Geometry: final body of the model. Coordinates: model frame, mm. Face numbers are marked on the shaded views. A direction names the side the tool comes from. Give positions to 0.01 mm unless a question says otherwise; leave off trailing zeros. Write each loop counter-clockwise with the first axis right and the second up, starting at its lowest first coordinate (ties: lowest second). Pieces come first, ordered by that corner, then holes. Notation, with made-up numbers: (-19.75, -23) -> (-9.75, -23) arc R11 ccw to (-9.75, -18) -> close; hole circle Ø4 at (59, 16.25). An arc over 180 degrees is marked (long way). Answer in a Markdown table with one row per item. Add a question column.
Item 1: Section query C-C on z = -28.5. Output: boundary loops of the cut face in (x, y).
Item 2: First-contact query: P1, Ø0.7, axis at x = -24.5, y = -7, coming from the +Z side; P2, Ø3, axis at x = -11.5, y = 2.5, coming from the -Z side; P3, Ø2, axis at x = 8, z = -39.5, coming from the +Y side. Flat tips, straight axial feed; report the tip coordinate or a pass-through.
Item 3: Material intervals for probe 1 along Y at (x, z) = (-13, -43); probe 2 along Z at (x, y) = (0, -6.25); probe 3 along Z at (x, y) = (11, 2), sorted ascending. Write a range as from..to.
Item 4: Section query A-A on y = -9. Output: boundary loops of the cut face in (x, z), plus the area to 3 significant figures.
Item 5: Access query for the marked faces 4, 5, 6, 7 and 8. Directions: +Z, -Z, +X, -X, +Y, -Y. A direction counts if a zero-diameter tool reaches every point of the face in a straight line with its end or side. Return the directions, or none.
Item 6: Section query D-D on x = 5.5. Output: boundary loops of the cut face in (y, z), plus the area to 3 significant figures.
Item 7: Draft query along X for the marked faces 1, 2 and 3. Return one class per face: +X half, -X half, draft (parallel to the pull), parting line (faces both ways), or undercut.
Item 8: Section query B-B on x = -3. Output: boundary loops of the cut face in (y, z).
```python
from build123d import *

# Parameters (mm, degrees)
BOSS_EXTRUDE1_DEPTH = 12.7
SKETCH1_5_W         = 47.483470806
SKETCH1_5_H         = 3.175
BOSS_EXTRUDE2_DEPTH = 6.35
SKETCH1_6_W         = 47.483470806
SKETCH1_6_H         = 3.175
BOSS_EXTRUDE3_DEPTH = 19.05


with BuildPart() as part:
    # Sketch1 → Boss-Extrude1 (new body)
    with BuildSketch(Plane(origin=(0, 0, 0), x_dir=(1, 0, 0), z_dir=(0, 1, 0))):
        with BuildLine():
            Line((25.211738376, 30.418429692), (33.470890643, 40.38325))
            ThreePointArc((33.470890643, 40.38325), (32.233303271, 41.377790676), (30.966181765, 42.334418478))
            Line((30.966181765, 42.334418478), (20.788013819, 41.890030069))
            Line((20.788013819, 41.890030069), (20.029841402, 40.059639939))
            Line((20.029841402, 40.059639939), (14.163206371, 42.489679735))
            Line((14.163206371, 42.489679735), (14.921378787, 44.320069864))
            Line((14.921378787, 44.320069864), (13.87332649, 50.582983434))
            ThreePointArc((13.87332649, 50.582983434), (0, 48.833429692), (-13.87332649, 50.582983434))
            Line((-13.87332649, 50.582983434), (-14.921378787, 44.320069864))
            Line((-14.921378787, 44.320069864), (-14.163206371, 42.489679735))
            Line((-14.163206371, 42.489679735), (-20.029841402, 40.059639939))
            Line((-20.029841402, 40.059639939), (-20.788013819, 41.890030069))
            Line((-20.788013819, 41.890030069), (-30.966181765, 42.334418478))
            ThreePointArc((-30.966181765, 42.334418478), (-32.233303271, 41.377790676), (-33.470890643, 40.38325))
            Line((-33.470890643, 40.38325), (-25.211738376, 30.418429692))
            Line((-25.211738376, 30.418429692), (25.211738376, 30.418429692))
        make_face()
    extrude(amount=-BOSS_EXTRUDE1_DEPTH)



with BuildPart() as body_2:
    # Sketch1<5> → Boss-Extrude2 (new body)
    with BuildSketch(Plane(origin=(0, 0, 0), x_dir=(1, 0, 0), z_dir=(0, 1, 0))):
        with Locations((0, 28.830929692)):
            Rectangle(SKETCH1_5_W, SKETCH1_5_H)
    extrude(amount=BOSS_EXTRUDE2_DEPTH)


with BuildPart() as part_1:
    add(part.part)

    add(body_2.part)  # Boss-Extrude3 merges body 2
    # Sketch1<6> → Boss-Extrude3 (add)
    with BuildSketch(Plane(origin=(0, 0, 0), x_dir=(1, 0, 0), z_dir=(0, 1, 0))):
        with Locations((0, 28.830929692)):
            Rectangle(SKETCH1_6_W, SKETCH1_6_H)
    extrude(amount=-BOSS_EXTRUDE3_DEPTH)


solid = part_1.part
```
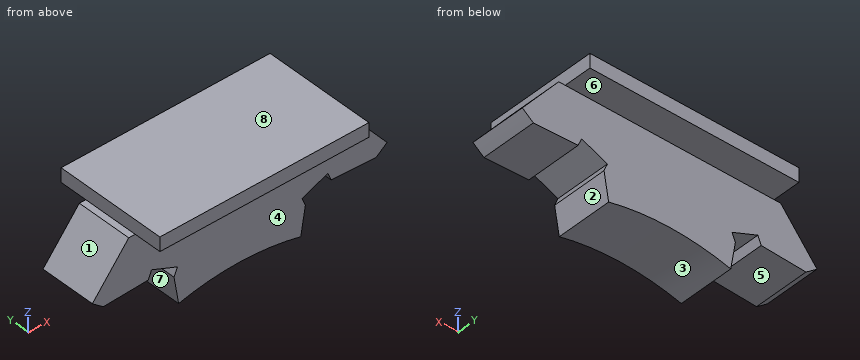
Findings below:
| question | item | result |
|---|---|---|
| 1 | outline | (-23.74, -19.05) -> (23.74, -19.05) -> (23.74, 6.35) -> (-23.74, 6.35) -> close |
| 2 | P1 | stops at z = -30.42 |
| 2 | P2 | stops at z = -30.42 |
| 2 | P3 | stops at y = 0 |
| 3 | probe 1 | y = -12.7..0 |
| 3 | probe 2 | z = -48.83..-27.24 |
| 3 | probe 3 | z = -30.42..-27.24 |
| 4 | outline | (-33.47, -40.38) arc R52.45 ccw to (-30.97, -42.33) -> (-20.79, -41.89) -> (-20.03, -40.06) -> (-14.16, -42.49) -> (-14.92, -44.32) -> (-13.87, -50.58) arc R55.88 cw to (13.87, -50.58) -> (14.92, -44.32) -> (14.16, -42.49) -> (20.03, -40.06) -> (20.79, -41.89) -> (30.97, -42.33) arc R52.45 ccw to (33.47, -40.38) -> (25.21, -30.42) -> (23.74, -30.42) -> (23.74, -27.24) -> (-23.74, -27.24) -> (-23.74, -30.42) -> (-25.21, -30.42) -> close |
| 4 | area | 1,050 mm^2 |
| 5 | face 4 | -Z, +X, -X, -Y |
| 5 | face 5 | -Z, +Y, -Y |
| 5 | face 6 | -Z, +X, -X, +Y |
| 5 | face 7 | -Z, -X, +Y, -Y |
| 5 | face 8 | +Z, +X, -X, +Y, -Y |
| 6 | outline | (-19.05, -30.42) -> (-12.7, -30.42) -> (-12.7, -49.1) -> (0, -49.1) -> (0, -30.42) -> (6.35, -30.42) -> (6.35, -27.24) -> (-19.05, -27.24) -> close |
| 6 | area | 318 mm^2 |
| 7 | face 1 | -X half |
| 7 | face 2 | +X half |
| 7 | face 3 | undercut |
| 8 | outline | (-19.05, -30.42) -> (-12.7, -30.42) -> (-12.7, -48.91) -> (0, -48.91) -> (0, -30.42) -> (6.35, -30.42) -> (6.35, -27.24) -> (-19.05, -27.24) -> close |
